Could you check a few things on this model? Use its own coordinates, in mm. Face numbers are marked on the shaded views. Round coordinates to 2 decimals unless told otherwise and drop trailing zeros. Loops run counter-clockwise (first coordinate to the right, second up) from the corner with the lowest first, then second, coordinate; pieces in that order, holes last. Notation, with made-up numbers: (14.25, 61) -> (45.25, 61) arc R18 ccw to (45.25, 70) -> close; hole circle Ø4 at (80, 84.5). An arc over 180 degrees is marked (long way). Use CSV: the item, a comma, the result in double quotes. Start each with the question number.
```python
from build123d import *

# Parameters (mm, degrees)
F0_R         = 65
F0_R_2       = 40
F1_DEPTH     = 350
F3_DEPTH     = 65.001
F5_DEPTH     = 65.0010001
F6_T4_DEPTH  = 251.2347538298
F6_S5_R      = 65
F6_T6_DEPTH  = 130
F6_S7_R      = 40
F6_T8_DEPTH  = 130
F6_T12_DEPTH = 251.2347538298
F6_S13_R     = 65
F6_T14_DEPTH = 130
F6_S15_R     = 40
F6_T16_DEPTH = 130
F8_DEPTH     = 65.0010001
F10_DEPTH    = 65.0010001


# Not quite as in the source:
# - a fillet or chamfer that OpenCascade refuses, or shapes differently, is made with other operations: its cross-section is extruded or revolved along the edge and cut away or added


with BuildPart() as f1:
    # F0 (on Front) → F1 (new body, symmetric)
    with BuildSketch(Plane.XZ):
        Circle(F0_R)
        Circle(F0_R_2, mode=Mode.SUBTRACT)
    extrude(amount=F1_DEPTH, both=True)

    # F2 (on Top) → F3 (cut, through all)
    with BuildSketch(Plane.XY):
        with BuildLine():
            ThreePointArc((-40, 160), (0, 120), (40, 160))
            ThreePointArc((40, 160), (0, 200), (-40, 160))
        make_face()
        with BuildLine():
            Line((40, 40), (40, 160))
            ThreePointArc((40, 160), (0, 120), (-40, 160))
            Line((-40, 160), (-40, -40))
            Line((-40, -40), (65, -40))
            Line((65, -40), (65, 40))
            Line((65, 40), (40, 40))
        make_face()
    extrude(amount=F3_DEPTH, mode=Mode.SUBTRACT)

    # F4 (on Right) → F5 (cut, through all)
    with BuildSketch(Plane.YZ):
        with BuildLine():
            ThreePointArc((-160, -40), (-131.7157287525, -28.2842712475), (-120, 0))
            ThreePointArc((-120, 0), (-131.7157287525, 28.2842712475), (-160, 40))
            ThreePointArc((-160, 40), (-200, 0), (-160, -40))
        make_face()
        with BuildLine():
            ThreePointArc((-160, 40), (-131.7157287525, 28.2842712475), (-120, 0))
            ThreePointArc((-120, 0), (-131.7157287525, -28.2842712475), (-160, -40))
            Line((-160, -40), (40, -40))
            Line((40, -40), (40, 65))
            Line((40, 65), (-40, 65))
            Line((-40, 65), (-40, 40))
            Line((-40, 40), (-160, 40))
        make_face()
    extrude(amount=F5_DEPTH, mode=Mode.SUBTRACT)

    # F6: fillet of radius 40 on 2 edges, made by hand


with BuildPart() as f6_tool2:
    # F6_s3 → F6_t4 (new body)
    with BuildSketch(Plane.YZ.offset(-100)):
        with BuildLine():
            ThreePointArc((0, -40), (28.2842712475, -28.2842712475), (40, 0))
            Line((40, 0), (40, -40))
            Line((40, -40), (0, -40))
        make_face()
    extrude(amount=F6_T4_DEPTH)

    # F6_s5 → F6_t6 (intersect, symmetric)
    with BuildSketch(Plane.XZ.offset(-20)):
        Circle(F6_S5_R)
    extrude(amount=F6_T6_DEPTH, both=True, mode=Mode.INTERSECT)

    # F6_s7 → F6_t8 (cut, symmetric)
    with BuildSketch(Plane.XZ.offset(-20)):
        Circle(F6_S7_R)
    extrude(amount=F6_T8_DEPTH, both=True, mode=Mode.SUBTRACT)


with BuildPart() as f1_1:
    add(f1.part)

    # F6_t1: union F6_tool2
    add(f6_tool2.part)


with BuildPart() as f6_tool10:
    # F6_s11 → F6_t12 (new body)
    with BuildSketch(Plane.XY.offset(-100)):
        with BuildLine():
            ThreePointArc((-40, 0), (-28.2842712475, -28.2842712475), (0, -40))
            Line((0, -40), (-40, -40))
            Line((-40, -40), (-40, 0))
        make_face()
    extrude(amount=F6_T12_DEPTH)

    # F6_s13 → F6_t14 (intersect, symmetric)
    with BuildSketch(Plane.XZ.offset(20)):
        Circle(F6_S13_R)
    extrude(amount=F6_T14_DEPTH, both=True, mode=Mode.INTERSECT)

    # F6_s15 → F6_t16 (cut, symmetric)
    with BuildSketch(Plane.XZ.offset(20)):
        Circle(F6_S15_R)
    extrude(amount=F6_T16_DEPTH, both=True, mode=Mode.SUBTRACT)


with BuildPart() as f1_2:
    add(f1_1.part)

    # F6_t9: union F6_tool10
    add(f6_tool10.part)

    # F7 (on Top) → F8 (cut, through all)
    with BuildSketch(Plane.XY):
        with BuildLine():
            ThreePointArc((11.2347538298, -40), (39.5190250773, -51.7157287525), (51.2347538298, -80))
            Line((51.2347538298, -80), (51.2347538298, -40))
            Line((51.2347538298, -40), (11.2347538298, -40))
        make_face()
    extrude(amount=F8_DEPTH, mode=Mode.SUBTRACT)

    # F9 (on Right) → F10 (cut, through all)
    with BuildSketch(Plane.YZ):
        with BuildLine():
            ThreePointArc((40, 11.2347538298), (51.7157287525, 39.5190250773), (80, 51.2347538298))
            Line((80, 51.2347538298), (40, 51.2347538298))
            Line((40, 51.2347538298), (40, 11.2347538298))
        make_face()
    extrude(amount=F10_DEPTH, mode=Mode.SUBTRACT)


solid = f1_2.part
```
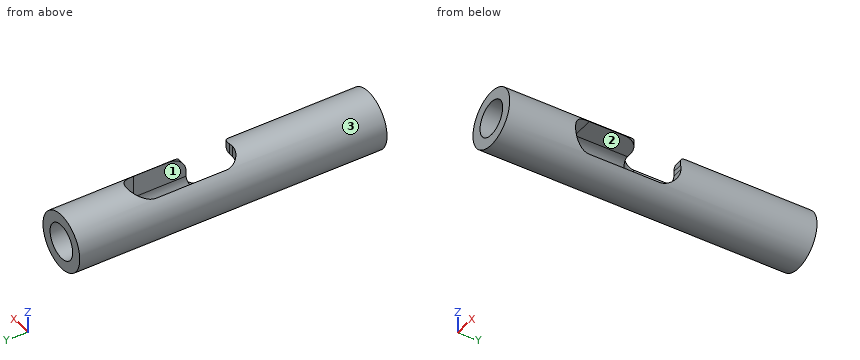
1. Suppose I cut it at C-C (y = 301). List the corners of the cut face in (x, z) for me, then the cut area to 3 significant figures.
2. If I drill on L1, parallel to Z at x = 3, y = -173; L2, parallel to Z at x = 2.5, y = 267.5; L3, parallel to Y at x = 35.5, z = 21.5, over which ranges is the centre line in solid material (lowest first)?
3. Will these pins go through, and if not, where does the flat tip stop? pin 1 (10 mm diameter, centred on y = 77, z = 28, fed in from +X); pin 2 (10 mm diameter, centred on x = 16, z = -30.5, fed in from -Y); pin 3 (10 mm diameter, centred on y = -33.5, z = -7.5, fed in from -X); pin 4 (12 mm diameter, centred on y = -205.5, z = 12, fed in from +X).
4. Suppose I cut it at B-B (x = 25.5). List the corners of the cut face in (y, z) for me.
5. Suppose I cut it at D-D (y = 51.5). List the corners of the cut face in (x, z) for me.
6. Suppose I cut it at A-A (z = -18.5). List the corners of the cut face in (x, y) for me.
7. We'd pull the mould along X, two halves only. Please class the marked faces 1, 2 and 3: pulls with the +X half, pulls with the -X half, needs draft (parallel to the pull), parting line crosses it, or undercut.
Geometry check:
1,outline,"circle Ø130 at (0, 0); hole circle Ø80 at (0, 0)"
1,area,"8,250 mm²"
2,L1,"z = -64.93 to -39.89, 39.89 to 64.93"
2,L2,"z = -64.95 to -39.92, 39.92 to 64.95"
2,L3,"y = -350 to -193.73, 178.43 to 350"
3,pin 1,"stops at x = 60.79"
3,pin 2,"passes through"
3,pin 3,"stops at x = -64.95"
3,pin 4,"stops at x = 64.72"
4,outline,"(-350, -59.79) -> (350, -59.79) -> (350, -30.82) -> (25.5, -30.82) arc R40 cw to (0, -40) -> (-160, -40) arc R40 cw to (-185.5, -30.82) -> (-350, -30.82) -> close; (-350, 30.82) -> (-185.5, 30.82) arc R40 cw to (-160, 40) -> (-42.63, 40) -> (-42.63, 59.79) -> (-350, 59.79) -> close; (190.82, 30.82) -> (350, 30.82) -> (350, 59.79) -> (190.82, 59.79) -> close"
5,outline,"(-40, 0) -> (-40, 51.23) arc R65 ccw (long way) to (51.77, 39.3) -> (40, 39.3) -> (40, 0) arc R40 cw to start"
6,outline,"(-62.31, -350) -> (-35.46, -350) -> (-35.46, 350) -> (-62.31, 350) -> close; (35.46, -350) -> (62.31, -350) -> (62.31, -195.46) -> (35.46, -195.46) -> close; (35.46, 35.46) -> (62.31, 35.46) -> (62.31, 350) -> (35.46, 350) -> close"
7,face 1,"undercut"
7,face 2,"needs draft"
7,face 3,"parting line crosses it"
